```python
from build123d import *

# Parameters (mm, degrees)
F0_W     = 994
F0_H     = 2000
F1_DEPTH = 18
F2_R     = 12.5
F3_DEPTH = 1
F4_W     = 450
F4_H     = 1000
F5_DEPTH = 82
F6_W     = 471.055174
F6_H     = 1022.924457
F6_W_2   = 450
F6_H_2   = 1000
F7_DEPTH = 82


with BuildPart() as f1:
    # F0 (on Front) → F1 (new body)
    with BuildSketch(Plane.XZ):
        Rectangle(F0_W, F0_H)
    extrude(amount=-F1_DEPTH)

    # F2 (on face) → F3 (cut)
    with BuildSketch(Plane.XZ):
        with Locations((-150, 625)):
            Circle(F2_R)
    extrude(amount=-F3_DEPTH, mode=Mode.SUBTRACT)

    # F4 (on face) → F5 (cut)
    with BuildSketch(Plane.XZ):
        with Locations((-227, -455)):
            Rectangle(F4_W, F4_H)
    extrude(amount=-F5_DEPTH, mode=Mode.SUBTRACT)

    # F6 (on face) → F7 (join)
    with BuildSketch(Plane.XZ):
        with Locations((-229.790854, -457.599444)):
            Rectangle(F6_W, F6_H)
        with Locations((-227, -455)):
            Rectangle(F6_W_2, F6_H_2, mode=Mode.SUBTRACT)
    extrude(amount=-F7_DEPTH)


solid = f1.part
```
Build history of the part. All positions in model axes, mm. A direction names the side the tool comes from. Round coordinates to 2 decimals unless told otherwise and drop trailing zeros. Loops run counter-clockwise (first coordinate to the right, second up) from the corner with the lowest first, then second, coordinate; pieces in that order, holes last. Notation, with made-up numbers: M 43,25.5 L 68,25.5 A22 ccw 68,53.5 Z; hole C -7.5,-15 d10. An arc over 180 degrees is marked long. Answer as CSV lines item,"result".
1. Cut at B-B on y = 33. Write the cut outline in (x, z), then the cut area to 3 significant figures.
Resolved:
outline,"M -465.32,-969.06 L 5.74,-969.06 L 5.74,53.86 L -465.32,53.86 Z; hole M -452,-955 L -2,-955 L -2,45 L -452,45 Z"
area,"31,900 mm²"
2. 3-axis set-ups, long thin cutter, end or side, ignore diameter. For faces 1 (the flat face through (-233, 50, -969.062)), 2 (the flat face through (-465.318, 50, -465)), 3 (the flat face through (-452, 40, -462)): which of +Z, -Z, +X, -X, +Y, -Y reach the whole face in a straight line?
Resolved:
face 1,"-Z, +X, -X, +Y"
face 2,"+Z, -Z, -X, +Y"
face 3,"+Y, -Y"
3. Two-plate mould, pull along X, no slides. Class faces 4 (the flat face through (103, 18, 236)), 5 (the flat face through (5.737, 50, -465)), 6 (the flat face through (-230, 40, 45)): released by +X, released by -X, zero draft, split by the parting line, or undercut.
Resolved:
face 4,"zero draft"
face 5,"released by +X"
face 6,"undercut"
4. Cut at A-A on z = -599.5. Write the cut outline in (x, y).
Resolved:
outline,"M -497,0 L -452,0 L -452,82 L -465.32,82 L -465.32,18 L -497,18 Z; M -2,0 L 497,0 L 497,18 L 5.74,18 L 5.74,82 L -2,82 Z"
5. Cut at D-D on z = 399. Write the cut outline in (x, y).
Resolved:
outline,"M -497,0 L 497,0 L 497,18 L -497,18 Z"
6. Wall check: probe 1 along Z at (x, y) = (-150, 0.5); probe 2 along X at (y, z) = (0.2, 625); probe 3 along Z at (x, y) = (-211, 37). Give the ranges that are in metal, low to high. Write a range as [from, to].
Resolved:
probe 1,"z = [-1000, -955], [45, 612.5], [637.5, 1000]"
probe 2,"x = [-497, -162.5], [-137.5, 497]"
probe 3,"z = [-969.06, -955], [45, 53.86]"
7. Cut at C-C on x = 60.5. Write the cut outline in (y, z), then the cut area to 3 significant figures.
Resolved:
outline,"M 0,-1000 L 18,-1000 L 18,1000 L 0,1000 Z"
area,"36,000 mm²"
8. Flat gauge pins, fed straight in: P1, Ø15, axis at x = -150, z = 625, coming from the -Y side; P2, Ø19, axis at x = -320, y = 39.5, coming from the -Z side; P3, Ø1.5, axis at x = 220, z = -205.5, coming from the +Y side; P4, Ø2, axis at x = 123, z = -590.5, coming from the -Y side. Where does each tip first touch, or does it go through?
Resolved:
P1,"stops at y = 1"
P2,"stops at z = -969.06"
P3,"stops at y = 18"
P4,"stops at y = 0"
